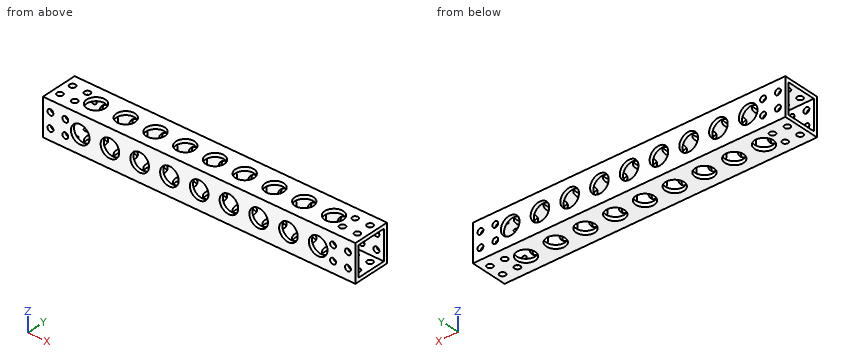
from build123d import *

# Parameters (mm, degrees)
SKETCH1_W           = 266.7
SKETCH1_H           = 31.75
BOSS_EXTRUDE1_DEPTH = 31.75
SKETCH2_R           = 7.9375
CUT_EXTRUDE1_DEPTH  = 31.75
LPATTERN1_COUNT     = 9
LPATTERN1_PITCH     = 25.4
SKETCH3_R           = 2.50825
CUT_EXTRUDE2_DEPTH  = 31.75
SKETCH4_W           = 25.4
SKETCH4_H           = 25.4
CUT_EXTRUDE3_DEPTH  = 266.7
SKETCH5_R           = 7.9375
CUT_EXTRUDE4_DEPTH  = 31.75
LPATTERN2_COUNT     = 9
LPATTERN2_PITCH     = 25.4
SKETCH6_R           = 2.50825
CUT_EXTRUDE5_DEPTH  = 31.75


with BuildPart() as part:
    # Sketch1 → Boss-Extrude1 (new body)
    with BuildSketch(Plane.XY):
        with Locations((-133.35, -15.875)):
            Rectangle(SKETCH1_W, SKETCH1_H)
    extrude(amount=BOSS_EXTRUDE1_DEPTH)

    # Sketch2 → Cut-Extrude1 (cut)
    with BuildSketch(Plane.XY.offset(31.75)):
        with Locations((-234.95, -15.875)):
            Circle(SKETCH2_R)
    cut_extrude1 = extrude(amount=-CUT_EXTRUDE1_DEPTH, mode=Mode.SUBTRACT)

    # LPattern1: Cut-Extrude1 ×9
    with Locations(*[(i * LPATTERN1_PITCH, 0, 0) for i in range(1, LPATTERN1_COUNT)]):
        add(cut_extrude1, mode=Mode.SUBTRACT)

    # Sketch3 → Cut-Extrude2 (cut)
    with BuildSketch(Plane.XY.offset(31.75)):
        with Locations((-260.35, -9.525)):
            Circle(SKETCH3_R)
        with Locations((-247.65, -9.525)):
            Circle(SKETCH3_R)
        with Locations((-260.35, -22.225)):
            Circle(SKETCH3_R)
        with Locations((-247.65, -22.225)):
            Circle(SKETCH3_R)
    cut_extrude2 = extrude(amount=-CUT_EXTRUDE2_DEPTH, mode=Mode.SUBTRACT)

    # Sketch4 → Cut-Extrude3 (cut)
    with BuildSketch(Plane(origin=(0, 0, 0), x_dir=(0, 0, -1), z_dir=(1, 0, 0))):
        with Locations((-15.875, -15.875)):
            Rectangle(SKETCH4_W, SKETCH4_H)
    extrude(amount=-CUT_EXTRUDE3_DEPTH, mode=Mode.SUBTRACT)

    # Mirror1: Cut-Extrude2 across plane
    add(cut_extrude2.mirror(Plane(origin=(-133.35, 0, 0), x_dir=(0, 0, 1), z_dir=(1, 0, 0))), mode=Mode.SUBTRACT)

    # Sketch5 → Cut-Extrude4 (cut)
    with BuildSketch(Plane(origin=(0, 0, 0), x_dir=(1, 0, 0), z_dir=(0, 1, 0))):
        with Locations((-31.75, -15.875)):
            Circle(SKETCH5_R)
    cut_extrude4 = extrude(amount=-CUT_EXTRUDE4_DEPTH, mode=Mode.SUBTRACT)

    # LPattern2: Cut-Extrude4 ×9
    with Locations(*[(-i * LPATTERN2_PITCH, 0, 0) for i in range(1, LPATTERN2_COUNT)]):
        add(cut_extrude4, mode=Mode.SUBTRACT)

    # Sketch6 → Cut-Extrude5 (cut)
    with BuildSketch(Plane(origin=(0, 0, 0), x_dir=(1, 0, 0), z_dir=(0, 1, 0))):
        with Locations((-19.05, -9.525)):
            Circle(SKETCH6_R)
        with Locations((-6.35, -9.525)):
            Circle(SKETCH6_R)
        with Locations((-19.05, -22.225)):
            Circle(SKETCH6_R)
        with Locations((-6.35, -22.225)):
            Circle(SKETCH6_R)
    cut_extrude5 = extrude(amount=-CUT_EXTRUDE5_DEPTH, mode=Mode.SUBTRACT)

    # Mirror2: Cut-Extrude5 across plane
    add(cut_extrude5.mirror(Plane(origin=(-133.35, 0, 0), x_dir=(0, 0, 1), z_dir=(1, 0, 0))), mode=Mode.SUBTRACT)


solid = part.part
Geometry check sheet. Reference: the model listing, model coordinates, mm. Round coordinates to 2 decimals unless told otherwise and drop trailing zeros. Loops run counter-clockwise (first coordinate to the right, second up) from the corner with the lowest first, then second, coordinate; pieces in that order, holes last.
Item 1: Cross-section at A-A on x = -184.15. Count the separate pieces of the cut face and the enclosed holes in it, then the cut area to 3 significant figures.
Item 2: Thickness scan on line 1 (Y direction, x = -232, z = 26.5) (3 decimals); line 2 (Y direction, x = -234.95, z = 31); line 3 (Z direction, x = -236.5, y = -24) (3 decimals). Record the ranges inside material, lowest first.
Item 3: Cross-section at C-C on x = -240.5. Record the boundary of the cut face in (y, z) (3 decimals), then the cut area to 3 significant figures.
Answer sheet:
1. separate pieces: 4
1. enclosed holes: 0
1. area: 161 mm2
2. line 1: y = -31.75 to -28.575, -3.175 to 0
2. line 2: y = -31.75 to -23.81, -7.94 to 0
2. line 3: z = 0 to 3.175, 28.575 to 31.75
3. outline: (-31.75, 0) - (-21.55, 0) - (-21.55, 3.175) - (-28.575, 3.175) - (-28.575, 10.2) - (-31.75, 10.2) - close; (-31.75, 21.55) - (-28.575, 21.55) - (-28.575, 28.575) - (-21.55, 28.575) - (-21.55, 31.75) - (-31.75, 31.75) - close; (-10.2, 0) - (0, 0) - (0, 10.2) - (-3.175, 10.2) - (-3.175, 3.175) - (-10.2, 3.175) - close; (-10.2, 28.575) - (-3.175, 28.575) - (-3.175, 21.55) - (0, 21.55) - (0, 31.75) - (-10.2, 31.75) - close
3. area: 219 mm2
